Could you check a few things on this drawing? It's one solid part, dimensions in mm from its lowest x, y, z. A direction names the side the tool comes from. Give positions to 0.01 mm unless a question says otherwise; leave off trailing zeros. Loops run counter-clockwise (first coordinate to the right, second up) from the corner with the lowest first, then second, coordinate; pieces in that order, holes last.
Q1. Thinking about a two-plate mould opening in X: for the marked faces 1, 2 and 3, which applies, pulls with the +X half, pulls with the -X half, needs draft (parallel to the pull), parting line crosses it, or undercut?
Q2. Suppose I cut it at C-C (y = 1.5). List the corners of the cut face in (x, z) for me (3 decimals), and give its area (3 significant figures).
Q3. Suppose I cut it at D-D (z = 6.5). List the corners of the cut face in (x, y) for me.
Q4. I'm going to push flat-ended pins straight in: P1, Ø1, axis at x = 4.5, z = 3, coming from the +Y side; P2, Ø1.9, axis at x = 5.5, y = 4.5, coming from the +Z side; P3, Ø3, axis at x = 2.5, z = 6, coming from the +Y side; P4, Ø1, axis at x = 1.5, z = 1.5, coming from the +Y side. Where does each tip first touch, or does it pass through?
Q5. I need wall thicknesses on probe 1 along Y at (x, z) = (5, 4.5); probe 2 along Z at (x, y) = (3.75, 4); probe 3 along Y at (x, z) = (4, 12.5). Which ranges of each line are inside material? Lowest first, please.
Q6. Suppose I cut it at B-B (x = 5). List the corners of the cut face in (y, z) for me (3 decimals), and give its area (3 significant figures).
Q7. Suppose I cut it at A-A (z = 13.75). List the corners of the cut face in (x, y) for me, and give its area (3 significant figures).
Q8. For the marked faces 4 and 5, which set-ups out of +Z, -Z, +X, -X, +Y, -Y let a thin tool reach every point of the face, with its end or its side?
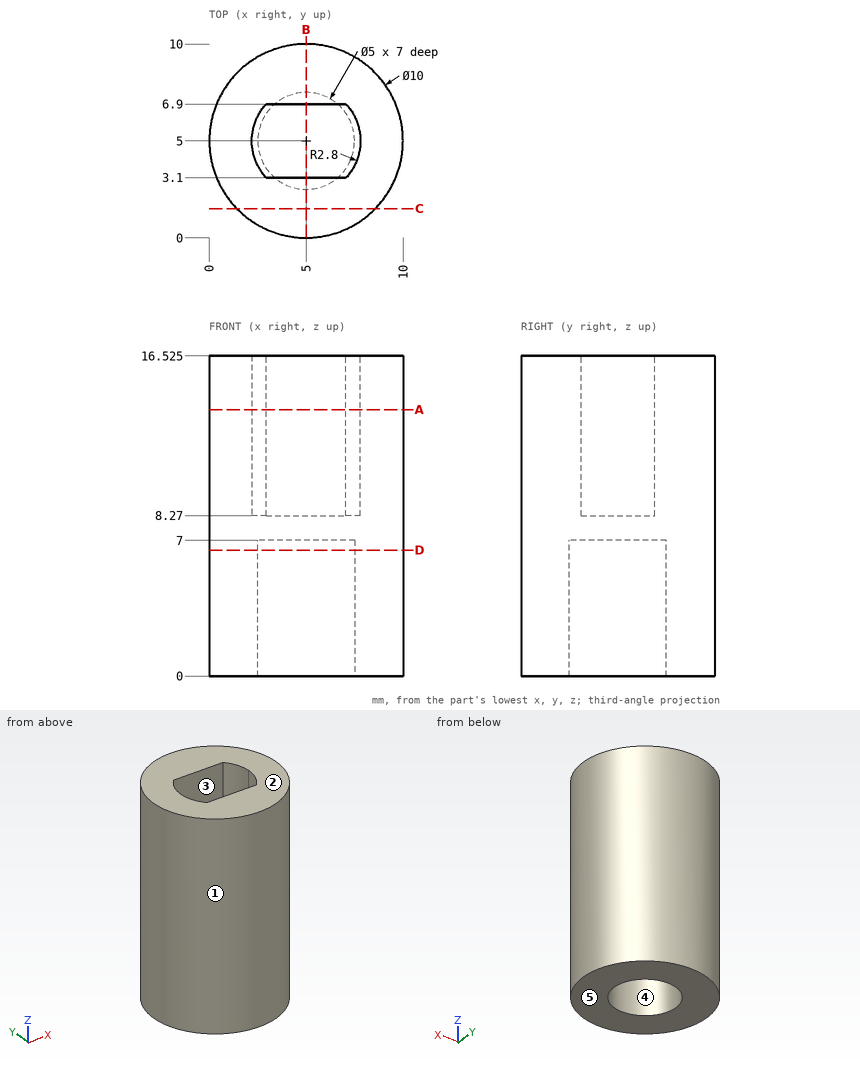
Solutions:
1. face 1: parting line crosses it
1. face 2: needs draft
1. face 3: undercut
2. outline: (1.429, 0) - (8.571, 0) - (8.571, 16.525) - (1.429, 16.525) - close
2. area: 118 mm2
3. outline: circle Ø10 at (5, 5); hole circle Ø5 at (5, 5)
4. P1: stops at y = 10
4. P2: stops at z = 8.27
4. P3: stops at y = 9.9
4. P4: stops at y = 9
5. probe 1: y = 0 to 2.5, 7.5 to 10
5. probe 2: z = 7 to 8.27
5. probe 3: y = 0.1 to 3.1, 6.9 to 9.9
6. outline: (0, 0) - (2.5, 0) - (2.5, 7) - (7.5, 7) - (7.5, 0) - (10, 0) - (10, 16.525) - (6.9, 16.525) - (6.9, 8.27) - (3.1, 8.27) - (3.1, 16.525) - (0, 16.525) - close
6. area: 98.9 mm2
7. outline: circle Ø10 at (5, 5); hole (2.94, 3.1) - (7.06, 3.1) arc R2.8 ccw to (7.8, 5) arc R2.8 ccw to (7.06, 6.9) - (2.94, 6.9) arc R2.8 ccw to start
7. area: 59.0 mm2
8. face 4: -Z
8. face 5: -Z, +X, -X, +Y, -Y
